from build123d import *

# Parameters (mm, degrees)
SKETCH2_W          = 16.237911894
SKETCH2_H          = 2
CUT_EXTRUDE1_DEPTH = 1


with BuildPart() as part:
    # Sketch1 → Revolve1 (revolve)
    with BuildSketch(Plane(origin=(0, 0, 0), x_dir=(1, 0, 0), z_dir=(0, 1, 0)), mode=Mode.PRIVATE) as revolve1_sk:
        Polygon((-3, -3), (0, -6), (0, 0), (-13, 0), (-11.845299462, -2), (-7.845299462, -2), (-7.845299462, -3), align=None)
    revolve(revolve1_sk.sketch.rotate(Axis((0, 0, 0), (-1, 0, 0)), 180), axis=Axis((0, 0, 0), (-1, 0, 0)))

    # Sketch2 → Cut-Extrude1 (cut)
    with BuildSketch(Plane(origin=(0, 0, 0), x_dir=(0, 0, -1), z_dir=(1, 0, 0))):
        Rectangle(SKETCH2_W, SKETCH2_H)
    extrude(amount=-CUT_EXTRUDE1_DEPTH, mode=Mode.SUBTRACT)


solid = part.part
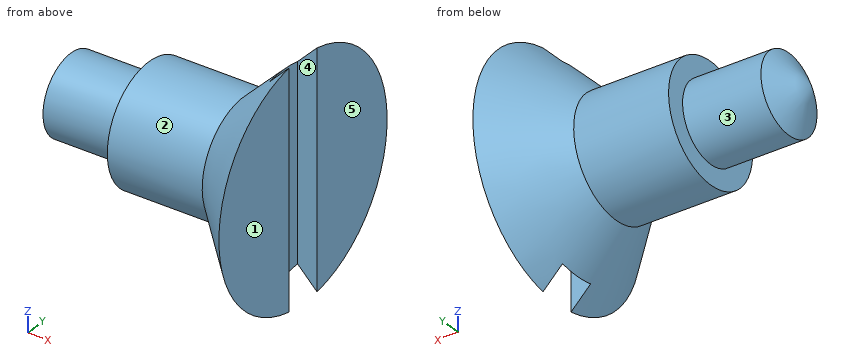
The listing builds one solid part. Answer for the finished solid, in the listing's coordinates (mm). Face numbers are marked on the shaded views. A direction names the side the tool comes from. Round coordinates to 2 decimals unless told otherwise and drop trailing zeros. Order: outer loops, then holes, each group sorted by start corner. A loop starts at its lowest first (then second) coordinate and runs counter-clockwise, first axis right, second up. Notation, with made-up numbers: M -17,-36 L 2,-36 A14 cw 2,-11 Z; hole C 73.5,31 d4. An arc over 180 degrees is marked long. Answer in a Markdown table with one row per item. Add a question column.
1) Consider line 1 along X through (y, z) = (0.25, 2.75); line 2 along X through (y, z) = (1.5, 1.5); line 3 along Y through (x, z) = (-4.5, 0). Determine where each line is inside the solid, lowest interval first. Write a range as from..to.
2) Flat-ended cylindrical pins translate along their axes: pin 1 Ø1 at (x, z) = (-9, 1) entering from +Y; pin 2 Ø3 at (y, z) = (-3.5, 1) entering from -X; pin 3 Ø0.5 at (x, z) = (-0.5, 1) entering from +Y. Find the tip coordinate at first contact, or state that the pin passes through.
3) The part is cut by section A-A on x = -7.5. Determine the outline of the cut face in (y, z).
4) Which of the six approach directions +Z, -Z, +X, -X, +Y, -Y give full straight-line access (tool end or side, diameter ignored) to the marked faces 1 and 2?
5) Determine the mould class of the marked faces 3, 4 and 5 for opening direction Y: pulls with the +Y half, pulls with the -Y half, needs draft (parallel to the pull), parting line crosses it, or undercut.
Findings below:
| question | item | result |
|---|---|---|
| 1 | line 1 | x = -7.85..-1 |
| 1 | line 2 | x = -7.85..0 |
| 1 | line 3 | y = -3..3 |
| 2 | pin 1 | stops at y = 1.94 |
| 2 | pin 2 | stops at x = -7.85 |
| 2 | pin 3 | stops at y = 5.67 |
| 3 | outline | C 0,0 d6 |
| 4 | face 1 | +Z, -Z, +X, +Y, -Y |
| 4 | face 2 | -X |
| 5 | face 3 | parting line crosses it |
| 5 | face 4 | undercut |
| 5 | face 5 | needs draft |
